Read the model definition and answer for the solid it produces. Units are mm, in the model's axes. Face numbers are marked on the shaded views. A direction names the side the tool comes from. Give positions to 0.01 mm unless a question says otherwise; leave off trailing zeros. Order: outer loops, then holes, each group sorted by start corner. A loop starts at its lowest first (then second) coordinate and runs counter-clockwise, first axis right, second up.
Item 1: A cutting plane is placed at D-D (y = -15). Write down the section's boundary in (x, z).
Item 2: Which of the six approach directions +Z, -Z, +X, -X, +Y, -Y give full straight-line access (tool end or side, diameter ignored) to the marked faces 1, 2 and 3?
Item 3: Find the intervals of material crossed by line 1 along X through (y, z) = (-131, 25.5); line 2 along Y through (x, z) = (-9, 21); line 3 along Z through (x, y) = (-50.5, -61.5), in increasing order.
Item 4: A cutting plane is placed at C-C (y = -98.5). Write down the section's boundary in (x, z), plus the area to 3 significant figures.
Item 5: The mould has two halves that part along X. Classify the marked faces 4, 5, 6 and 7: +X half, -X half, draft (parallel to the pull), parting line (faces both ways), or undercut.
Item 6: Given pin 1 Ø0.6 at (x, z) = (-56, 30) entering from -Y; pin 2 Ø3 at (x, z) = (20, 9.5) entering from -Y; pin 3 Ø4 at (y, z) = (19, 17.5) entering from -X, each flat-ended and moving along its own axis, determine where each tip first touches the part or whether it passes through.
Item 7: A cutting plane is placed at B-B (z = 34). Write down the section's boundary in (x, y), plus the area to 3 significant figures.
Item 8: A cutting plane is placed at A-A (x = 4). Write down the section's boundary in (y, z).
from build123d import *

# Parameters (mm, degrees)
SKETCH_1_W          = 110
SKETCH_1_H          = 150
EXTRUDE_1_DEPTH     = 3
SKETCH_2_W          = 110
SKETCH_2_H          = 150
SKETCH_2_W_2        = 104
SKETCH_2_H_2        = 144
EXTRUDE_2_DEPTH     = 20
EXTRUDE_3_DEPTH     = 20
SKETCH_4_W          = 41
SKETCH_4_H          = 20.685891883
EXTRUDE_4_DEPTH     = 2
SKETCH_5_W          = 70
SKETCH_5_H          = 15
CUT_EXTRUDE_1_DEPTH = 8
FILLET_1_R          = 5


with BuildPart() as part:
    # 草图1 → 凸台-拉伸1 (new body)
    with BuildSketch(Plane.XY):
        Rectangle(SKETCH_1_W, SKETCH_1_H)
    extrude(amount=EXTRUDE_1_DEPTH)

    # 草图2 → 凸台-拉伸2 (add)
    with BuildSketch(Plane.XY.offset(3)):
        Rectangle(SKETCH_2_W, SKETCH_2_H)
        Rectangle(SKETCH_2_W_2, SKETCH_2_H_2, mode=Mode.SUBTRACT)
    extrude(amount=EXTRUDE_2_DEPTH)

    # 草图3 → 凸台-拉伸3 (add)
    with BuildSketch(Plane.ZY.offset(55)):
        Polygon((23, -75), (38, -75), (38, -59.816209212), (41, -59.816209212), (41, -117.234969842), (5.700174456, -181.163787756), (0, -181.163787756), (0, -75), align=None)
    extrude_3 = extrude(amount=-EXTRUDE_3_DEPTH)

    # 草图4 → 凸台-拉伸4 (add)
    with BuildSketch(Plane.ZY.offset(55)):
        with Locations((20.5, -70.159155153)):
            Rectangle(SKETCH_4_W, SKETCH_4_H)
    extrude_4 = extrude(amount=EXTRUDE_4_DEPTH)

    # 草图5 → 切除-拉伸1 (cut)
    with BuildSketch(Plane(origin=(0, 75, 0), x_dir=(1, 0, 0), z_dir=(0, 1, 0))):
        with Locations((0, -10.5)):
            Rectangle(SKETCH_5_W, SKETCH_5_H)
    extrude(amount=-CUT_EXTRUDE_1_DEPTH, mode=Mode.SUBTRACT)

    # 圆角1
    fillet_1_edges = [part.edges().sort_by_distance(p)[0] for p in [
        (-35, 73.5, 18),
        (-35, 73.5, 3),
        (35, 73.5, 3),
        (35, 73.5, 18),
    ]]
    fillet(fillet_1_edges, radius=FILLET_1_R)

    # 镜向1: 凸台-拉伸4 across plane
    add(extrude_4.mirror(Plane(origin=(0, 0, 0), x_dir=(0, 0, 1), z_dir=(1, 0, 0))))

    # 镜向2: 凸台-拉伸3 across plane
    add(extrude_3.mirror(Plane(origin=(0, 0, 0), x_dir=(0, 0, 1), z_dir=(1, 0, 0))))


solid = part.part
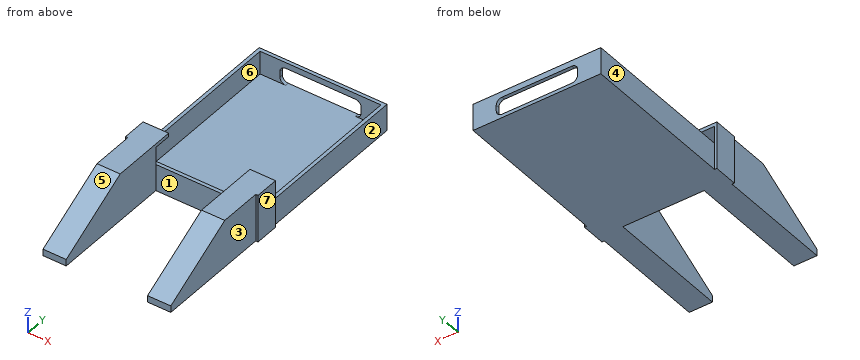
Response values:
1. outline: (-55, 0) - (55, 0) - (55, 23) - (52, 23) - (52, 3) - (-52, 3) - (-52, 23) - (-55, 23) - close
2. face 1: +Z, -Z, -Y
2. face 2: +Z, -Z, +X, +Y
2. face 3: +Z, -Z, +X, -Y
3. line 1: x = -55 to -35, 35 to 55
3. line 2: y = -75 to -72, 72 to 75
3. line 3: z = 0 to 3, 38 to 41
4. outline: (-55, 0) - (-35, 0) - (-35, 41) - (-55, 41) - close; (35, 0) - (55, 0) - (55, 41) - (35, 41) - close
4. area: 1,640 mm2
5. face 4: -X half
5. face 5: draft
5. face 6: undercut
5. face 7: +X half
6. pin 1: stops at y = -80.5
6. pin 2: stops at y = -75
6. pin 3: stops at x = -55
7. outline: (-57, -80.5) - (-55, -80.5) - (-55, -129.91) - (-35, -129.91) - (-35, -75) - (-55, -75) - (-55, -59.82) - (-57, -59.82) - close; (35, -129.91) - (55, -129.91) - (55, -80.5) - (57, -80.5) - (57, -59.82) - (55, -59.82) - (55, -75) - (35, -75) - close
7. area: 2,280 mm2
8. outline: (-75, 0) - (75, 0) - (75, 3) - (-72, 3) - (-72, 23) - (-75, 23) - close; (72, 18) - (75, 18) - (75, 23) - (72, 23) - close
